Model file for the job. Use its own axes, mm. Round coordinates to 2 decimals unless told otherwise and drop trailing zeros. Order: outer loops, then holes, each group sorted by start corner. A loop starts at its lowest first (then second) coordinate and runs counter-clockwise, first axis right, second up. Notation, with made-up numbers: (-18, 84.5) -> (5, 84.5) arc R27 cw to (5, 108.5) -> close; hole circle Ø3 at (-16.75, -26). An arc over 180 degrees is marked (long way). Answer as CSV lines item,"result".
Autodesk Inventor part; units mm, degrees
ref_plane "YZ Plane" through (0, 0, 0) normal (1, 0, 0) x (0, 1, 0)
ref_plane "XZ Plane" through (0, 0, 0) normal (0, 1, 0) x (-1, 0, 0)
ref_plane "XY Plane" through (0, 0, 0) normal (0, 0, 1) x (1, 0, 0)
sketch "Sketch1" plane through (0, 0, 0) normal (0, 1, 0) x (-1, 0, 0)
  circle A0 centre (17.2567, 94.6354) radius 6.35
  line L0 (22.3367, 94.6354) -> (12.1767, 94.6354)
  line L1 (12.1767, 94.6354) -> (12.1767, 18.4354)
  line L2 (12.1767, 18.4354) -> (22.3367, 18.4354)
  line L3 (22.3367, 18.4354) -> (22.3367, 94.6354)
  point P0 (0, 0)
  dimension "d0" = 12.7
  dimension "d1" = 76.2
  dimension "d2" = 0
  dimension "d3" = 10.16
  dimension "d4" = 5.08
extrude "Extrusion1" add sketch "Sketch1" along normal blind 101.6
sketch "Sketch2" plane through (0, 101.6, 0) normal (0, 1, 0) x (1, 0, 0)
  arc A0 (-22.3367, -90.8254) -> (-12.1767, -90.8254) centre (-17.2567, -94.6354) ccw
  circle A1 centre (-17.2567, -94.6354) radius 2.54
  point P0 (0, 0)
  dimension "d7" = 5.08
extrude "Extrusion2" cut sketch "Sketch2" against normal blind 482.6
sketch "Sketch3" plane through (0, 101.6, 0) normal (0, 1, 0) x (1, 0, 0)
  circle A0 centre (-17.2567, -26.0554) radius 2.8969
  line L0 (-12.1767, -18.4354) -> (-22.3367, -18.4354)
  line L1 (-22.3367, -18.4354) -> (-22.3367, -90.8254)
  point P0 (0, 0)
  dimension "d10" = 7.62
  dimension "d11" = 5.08
extrude "Extrusion3" cut sketch "Sketch3" against normal blind 482.6
sketch "Sketch4" plane through (0, 101.6, 0) normal (0, 1, 0) x (1, 0, 0)
  circle A0 centre (-17.2567, -33.6754) radius 2.6633
  line L0 (-12.1767, -90.8254) -> (-12.1767, -18.4354)
  line L1 (-12.1767, -18.4354) -> (-22.3367, -18.4354)
  point P0 (0, 0)
  dimension "d14" = 5.08
  dimension "d15" = 15.24
hole "Hole1" at (-17.2567, 101.6, 33.6754) direction (0, -1, 0) diameter 1.778 end through all
properties part number "Gripper"
Q1. Flat gauge pins, fed straight in: pin 1 (21.5 mm diameter, centred on y = 25.5, z = 37.5, fed in from -X); pin 2 (3.5 mm diameter, centred on x = -17.26, z = 26.06, fed in from -Y); pin 3 (21.5 mm diameter, centred on y = 51, z = 56, fed in from +X); pin 4 (1.5 mm diameter, centred on x = -15.5, y = 65.5, fed in from +Z). Where does each tip first touch, or does it go through?
Checks:
pin 1,"x = -22.34"
pin 2,"through"
pin 3,"x = -12.18"
pin 4,"z = 100.91"
Q2. Saw through at A-A (y = 64.5). Write the cut outline in (x, z).
Checks:
outline,"(-22.34, 18.44) -> (-12.18, 18.44) -> (-12.18, 90.83) arc R6.35 ccw (long way) to (-22.34, 90.83) -> close; hole circle Ø5.79 at (-17.26, 26.06); hole circle Ø5.08 at (-17.26, 94.64); hole circle Ø1.78 at (-17.26, 33.68)"
Q3. Mould opens along X. For faces 1 (the cylindrical face through (-19.392, 51.511, 24.098)), 2 (the flat face through (-17, 101.6, 60)), 3 (the flat face through (-22.337, 50, 54)), 4 (the flat face through (-12.177, 50, 55)) say: +X half, -X half, draft (parallel to the pull), parting line (faces both ways), or undercut.
Checks:
face 1,"undercut"
face 2,"draft"
face 3,"-X half"
face 4,"+X half"
Q4. Wall check: L1, parallel to Z at x = -18.25, y = 92; L2, parallel to Z at x = -19.5, y = 23.5; L3, parallel to Z at x = -16.75, y = 12. Give the ranges that are in metal, low to high. Write a range as [from, to].
Checks:
L1,"[18.44, 23.33], [28.78, 92.3], [96.97, 100.91]"
L2,"[18.44, 24.22], [27.89, 93.44], [95.83, 100.58]"
L3,"[18.44, 23.2], [28.91, 32.94], [34.41, 92.15], [97.12, 100.97]"
Q5. Saw through at B-B (z = 56.5). Write the cut outline in (x, y).
Checks:
outline,"(-22.34, 0) -> (-12.18, 0) -> (-12.18, 101.6) -> (-22.34, 101.6) -> close"
